Here's how the part is built. I have some questions about the finished solid (model axes, mm). Coordinates: 2 decimals unless noted, no trailing zeros. Use one line per item in the form item = value. Start each with the question number.
(1) Please list where these lines run through material, in increasing order: L1, parallel to X at y = 0.8, z = 9.5; L2, parallel to Z at x = -7.5, y = 1.75; L3, parallel to Z at x = -17, y = 2.1.
(2) Will these pins go through, and if not, where does the flat tip stop? P1, Ø5, axis at x = 62.69, z = 62.69, coming from the +Y side; P2, Ø2, axis at y = 1.5, z = -8.5, coming from the -X side; P3, Ø7, axis at x = -62.69, z = -62.69, coming from the +Y side.
(3) Imagine slicing it at A-A, the plane x = 0. State how many separate pieces and enclosed holes the cut face has, and give its area (3 significant figures).
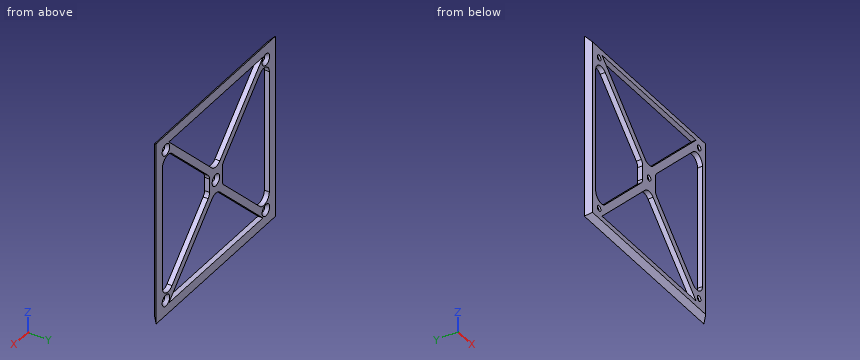
```python
from build123d import *

# Parameters (mm, degrees)
SKETCH1_W                                      = 150
SKETCH1_H                                      = 150
BOSS_EXTRUDE2_DEPTH                            = 4
CSK_FOR_M4_FLAT_HEAD_MACHINE_SCREW1_AT_2_COUNT = 2
CSK_FOR_M4_FLAT_HEAD_MACHINE_SCREW1_AT_2_PITCH = 88.653975713
CSK_FOR_M4_FLAT_HEAD_MACHINE_SCREW1_AT_3_COUNT = 2
CSK_FOR_M4_FLAT_HEAD_MACHINE_SCREW1_AT_3_PITCH = 88.653975713
CSK_FOR_M4_FLAT_HEAD_MACHINE_SCREW1_AT_4_COUNT = 2
CSK_FOR_M4_FLAT_HEAD_MACHINE_SCREW1_AT_4_PITCH = 88.653975713
CSK_FOR_M4_FLAT_HEAD_MACHINE_SCREW1_AT_5_COUNT = 2
CSK_FOR_M4_FLAT_HEAD_MACHINE_SCREW1_AT_5_PITCH = 88.653975713
CHAMFER2_SIZE                                  = 4


with BuildPart() as part:
    # Sketch1 → Boss-Extrude2 (new body)
    with BuildSketch(Plane(origin=(0, 0, 0), x_dir=(1, 0, 0), z_dir=(0, 1, 0))):
        Rectangle(SKETCH1_W, SKETCH1_H)
        with BuildLine():
            Line((-59, 67), (59, 67))
            Line((59, 67), (4.949747468, 12.949747468))
            ThreePointArc((4.949747468, 12.949747468), (0, 10.899494937), (-4.949747468, 12.949747468))
            Line((-4.949747468, 12.949747468), (-59, 67))
        make_face(mode=Mode.SUBTRACT)
        with BuildLine():
            Line((59, -67), (-59, -67))
            Line((-59, -67), (-4.949747468, -12.949747468))
            ThreePointArc((-4.949747468, -12.949747468), (0, -10.899494937), (4.949747468, -12.949747468))
            Line((4.949747468, -12.949747468), (59, -67))
        make_face(mode=Mode.SUBTRACT)
        with BuildLine():
            Line((-67, -50.100505063), (-67, 50.100505063))
            ThreePointArc((-67, 50.100505063), (-62.678784027, 56.567661791), (-55.050252532, 55.050252532))
            Line((-55.050252532, 55.050252532), (-9.757359313, 9.757359313))
            ThreePointArc((-9.757359313, 9.757359313), (-8.456722805, 7.81081922), (-8, 5.514718626))
            Line((-8, 5.514718626), (-8, -5.514718626))
            ThreePointArc((-8, -5.514718626), (-8.456722805, -7.81081922), (-9.757359313, -9.757359313))
            Line((-9.757359313, -9.757359313), (-55.050252532, -55.050252532))
            ThreePointArc((-55.050252532, -55.050252532), (-62.678784027, -56.567661791), (-67, -50.100505063))
        make_face(mode=Mode.SUBTRACT)
        with BuildLine():
            ThreePointArc((67, -50.100505063), (62.678784027, -56.567661791), (55.050252532, -55.050252532))
            Line((55.050252532, -55.050252532), (9.757359313, -9.757359313))
            ThreePointArc((9.757359313, -9.757359313), (8.456722805, -7.81081922), (8, -5.514718626))
            Line((8, -5.514718626), (8, 5.514718626))
            ThreePointArc((8, 5.514718626), (8.456722805, 7.81081922), (9.757359313, 9.757359313))
            Line((9.757359313, 9.757359313), (55.050252532, 55.050252532))
            ThreePointArc((55.050252532, 55.050252532), (62.678784027, 56.567661791), (67, 50.100505063))
            Line((67, 50.100505063), (67, -50.100505063))
        make_face(mode=Mode.SUBTRACT)
    extrude(amount=BOSS_EXTRUDE2_DEPTH)

    # Sketch5 → CSK for M4 Flat Head Machine Screw1 (revolve, cut)
    with BuildSketch(Plane(origin=(0, 4, 0), x_dir=(0, 0, 1), z_dir=(1, 0, 0))):
        Polygon((0, 0), (0, 4), (2.25, 4), (2.25, 2.45), (4.7, 0), align=None)
    csk_for_m4_flat_head_machine_screw1 = revolve(axis=Axis((0, 10.35, 0), (0, -1, 0)), mode=Mode.SUBTRACT)

    # CSK for M4 Flat Head Machine Screw1 at 2: CSK for M4 Flat Head Machine Screw1 ×2
    with Locations(*[Vector(-0.7071067811865477, 0, -0.7071067811865474) * (i * CSK_FOR_M4_FLAT_HEAD_MACHINE_SCREW1_AT_2_PITCH) for i in range(1, CSK_FOR_M4_FLAT_HEAD_MACHINE_SCREW1_AT_2_COUNT)]):
        add(csk_for_m4_flat_head_machine_screw1, mode=Mode.SUBTRACT)

    # CSK for M4 Flat Head Machine Screw1 at 3: CSK for M4 Flat Head Machine Screw1 ×2
    with Locations(*[Vector(0.7071067811865477, 0, -0.7071067811865474) * (i * CSK_FOR_M4_FLAT_HEAD_MACHINE_SCREW1_AT_3_PITCH) for i in range(1, CSK_FOR_M4_FLAT_HEAD_MACHINE_SCREW1_AT_3_COUNT)]):
        add(csk_for_m4_flat_head_machine_screw1, mode=Mode.SUBTRACT)

    # CSK for M4 Flat Head Machine Screw1 at 4: CSK for M4 Flat Head Machine Screw1 ×2
    with Locations(*[Vector(0.7071067811865477, 0, 0.7071067811865474) * (i * CSK_FOR_M4_FLAT_HEAD_MACHINE_SCREW1_AT_4_PITCH) for i in range(1, CSK_FOR_M4_FLAT_HEAD_MACHINE_SCREW1_AT_4_COUNT)]):
        add(csk_for_m4_flat_head_machine_screw1, mode=Mode.SUBTRACT)

    # CSK for M4 Flat Head Machine Screw1 at 5: CSK for M4 Flat Head Machine Screw1 ×2
    with Locations(*[Vector(-0.7071067811865477, 0, 0.7071067811865474) * (i * CSK_FOR_M4_FLAT_HEAD_MACHINE_SCREW1_AT_5_PITCH) for i in range(1, CSK_FOR_M4_FLAT_HEAD_MACHINE_SCREW1_AT_5_COUNT)]):
        add(csk_for_m4_flat_head_machine_screw1, mode=Mode.SUBTRACT)

    # Chamfer2
    chamfer2_edges = [part.edges().sort_by_distance(p)[0] for p in [
        (0, 0, 75),
        (-75, 0, 0),
        (0, 0, -75),
        (75, 0, 0),
    ]]
    chamfer(chamfer2_edges, length=CHAMFER2_SIZE - 0.0001)  # a hair under: the kernel refuses the full size


solid = part.part
```
Answer:
q1.L1 = -71.8 to -67, -9.51 to 9.51, 67 to 71.8
q1.L2 = -72.75 to -67, -15.5 to 15.5, 67 to 72.75
q1.L3 = -73.1 to -67, -25 to -17, 17 to 25, 67 to 73.1
q2.P1 = 1.8
q2.P2 = -73.5
q2.P3 = 2.8
q3.separate_pieces = 4
q3.enclosed_holes = 0
q3.area = 111 mm²
